Verification items for the finished model (mm, model axes). A direction names the side the tool comes from. Coordinates: 2 decimals unless noted, no trailing zeros. Write each loop counter-clockwise with the first axis right and the second up, starting at its lowest first coordinate (ties: lowest second). Pieces come first, ordered by that corner, then holes. Notation, with made-up numbers: (43, -38) -> (73, -38) arc R4 ccw to (73, -33) -> close; hole circle Ø1 at (-13.5, 88). An arc over 180 degrees is marked (long way). Use CSV: the item, a comma, the result in double quotes.
```python
from build123d import *

# Parameters (mm, degrees)
L_ANGLE_EQUAL_60X60X6_3_DEPTH = 1570
SKETCH14_R                    = 8
CUT_EXTRUDE1_DEPTH            = 1573.291321607


with BuildPart() as part:
    # Sketch17 → L angle (equal) 60X60X6(3) (new body)
    with BuildSketch(Plane(origin=(0, 0, 0), x_dir=(0, 0, -1), z_dir=(1, 0, 0))):
        with BuildLine():
            Line((0, 60), (0, 0))
            Line((0, 0), (60, 0))
            ThreePointArc((60, 0), (58.242640687, 4.242640687), (54, 6))
            Line((54, 6), (14, 6))
            ThreePointArc((14, 6), (8.343145751, 8.343145751), (6, 14))
            Line((6, 14), (6, 54))
            ThreePointArc((6, 54), (4.242640687, 58.242640687), (0, 60))
        make_face()
    extrude(amount=L_ANGLE_EQUAL_60X60X6_3_DEPTH)

    # Sketch14 → Cut-Extrude1 (cut, through all)
    with BuildSketch(Plane.XY):
        with Locations((285, 30)):
            Circle(SKETCH14_R)
        with Locations((1285, 30)):
            Circle(SKETCH14_R)
        Polygon((1570, 0), (1570, 60), (1510, 60), align=None)
        Polygon((0, 60), (0, 0), (60, 60), align=None)
    extrude(amount=-CUT_EXTRUDE1_DEPTH, mode=Mode.SUBTRACT)


solid = part.part
```
1) Cross-section at A-A (x = 1430.5). Record the boundary of the cut face in (y, z).
Return value:
outline,"(0, -60) arc R6 ccw to (6, -54) -> (6, -14) arc R8 cw to (14, -6) -> (54, -6) arc R6 ccw to (60, 0) -> (0, 0) -> close"
2) Cross-section at B-B (z = -35). Record the boundary of the cut face in (x, y).
Return value:
outline,"(0, 0) -> (1570, 0) -> (1564, 6) -> (6, 6) -> close"
3) Scan lines: L1, parallel to Y at x = 285, z = -1.5; L2, parallel to Z at x = 983, y = 54.5; L3, parallel to Y at x = 252.5, z = -46.5. Record each from-to range of solid material in increasing order.
Return value:
L1,"0 to 22, 38 to 59.81"
L2,"-5.98 to 0"
L3,"0 to 6"
4) Set-up check for faces 1 (the flat face through (17, 17, -5)), 2 (the flat face through (774, 6, -34)): record each of +Z, -Z, +X, -X, +Y, -Y from which the full face is reachable in a straight line by a thin tool's end or side.
Return value:
face 1,"+Z, -Z, -X, +Y"
face 2,"-Z, +X, -X, +Y"
5) Gauge pin test, flat ends, axial feed: pin 1 (2 mm diameter, centred on x = 1031.5, y = 23.5, fed in from -Z); pin 2 (1 mm diameter, centred on x = 1403.5, z = -19, fed in from +Y). Record the tip position at first contact, or that the pin passes through.
Return value:
pin 1,"z = -6"
pin 2,"y = 6"
